Can you work these out from the model? Positions are in its coordinate system, mm. Face numbers are marked on the shaded views. Give positions to 0.01 mm unless a question says otherwise; leave off trailing zeros. Order: outer loops, then holes, each group sorted by start corner. A loop starts at its lowest first (then second) coordinate and runs counter-clockwise, first axis right, second up. Notation, with made-up numbers: (80, 61.25) - (100, 61.25) arc R27 ccw to (100, 77.25) - close; hole circle Ø7 at (3, 71.25). An arc over 180 degrees is marked (long way). Use one line per item in the form item = value. Start each with the question number.
1) Please list where these lines run through material, in increasing order: probe 1 along X at (y, z) = (51, 0); probe 2 along X at (y, z) = (15, -4.5); probe 3 along Z at (x, y) = (8, 77.5).
2) Suppose I cut it at A-A, the plane x = 0. Write out the boundary of the cut face in (y, z), and give its area (3 significant figures).
3) We'd pull the mould along Z, two halves only. Please class the marked faces 1 and 2: released by +Z, released by -Z, zero draft, split by the parting line, or undercut.
4) Suppose I cut it at B-B, the plane z = 0. Write out the boundary of the cut face in (x, y), and give its area (3 significant figures).
5) Suppose I cut it at C-C, the plane y = 51. Write out the boundary of the cut face in (x, z), and give its area (3 significant figures).
6) For pin 1 (12 mm diameter, centred on x = -18.5, y = 81, fed in from +Z); pin 2 (5 mm diameter, centred on y = 36, z = -9, fed in from -X); pin 3 (3 mm diameter, centred on x = -11, y = 34, fed in from +Z), each with a flat end and sliding along its axis, tell me the tip position at first contact or that it passes through.
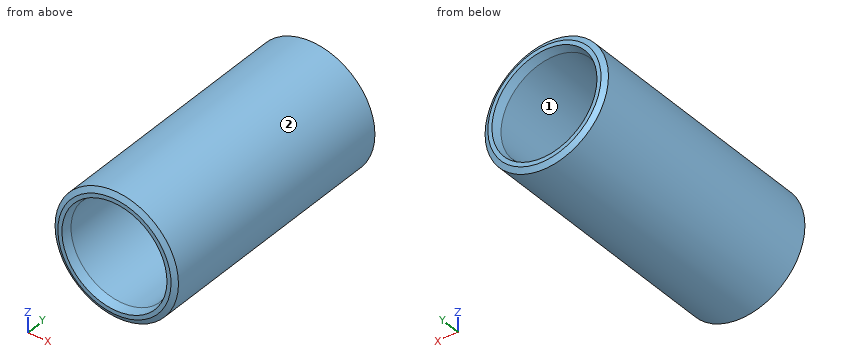
```python
from build123d import *

# Parameters (mm, degrees)
DURCHMESSER_WD_R   = 24.15
DURCHMESSER_WD_R_2 = 19.65
ROHR_DEPTH         = 100


with BuildPart() as part:
    # Durchmesser/ WD → Rohr (new body)
    with BuildSketch(Plane(origin=(0, 0, 0), x_dir=(1, 0, 0), z_dir=(0, 1, 0))):
        with Locations(Location((0, 0, 0), (0, 0, 270))):  # turned: the seam where the file's is
            Circle(DURCHMESSER_WD_R)
        with Locations(Location((0, 0, 0), (0, 0, 270))):  # turned: the seam where the file's is
            Circle(DURCHMESSER_WD_R_2, mode=Mode.SUBTRACT)
    extrude(amount=ROHR_DEPTH)

    # Fase1 → Schweißfase 1 (revolve, cut)
    with BuildSketch(Plane.XY, mode=Mode.PRIVATE) as schwei_fase_1_sk:
        Polygon((24.15, 100), (24.15, 98.845299462), (22.15, 100), align=None)
        Polygon((20.55, 100), (19.65, 100), (19.65, 96.641154273), align=None)
    revolve(schwei_fase_1_sk.sketch.rotate(Axis((0, 0, 0), (0, 1, 0)), 90), axis=Axis((0, 0, 0), (0, 1, 0)), mode=Mode.SUBTRACT)  # turned: the seam where the file's is

    # Fase2 → Schweißfase 2 (revolve, cut)
    with BuildSketch(Plane.XY, mode=Mode.PRIVATE) as schwei_fase_2_sk:
        Polygon((24.15, 0), (24.15, 1.154700538), (22.15, 0), align=None)
        Polygon((20.55, 0), (19.65, 0), (19.65, 3.358845727), align=None)
    revolve(schwei_fase_2_sk.sketch.rotate(Axis((0, 0, 0), (0, 1, 0)), 90), axis=Axis((0, 0, 0), (0, 1, 0)), mode=Mode.SUBTRACT)  # turned: the seam where the file's is


solid = part.part
```
Result sheet:
q1.probe_1 = -24.15 to -19.65, 19.65 to 24.15
q1.probe_2 = -23.73 to -19.13, 19.13 to 23.73
q1.probe_3 = -22.79 to -17.95, 17.95 to 22.79
q2.outline = (0, -22.15) - (1.15, -24.15) - (98.85, -24.15) - (100, -22.15) - (100, -20.55) - (96.64, -19.65) - (3.36, -19.65) - (0, -20.55) - close; (0, 20.55) - (3.36, 19.65) - (96.64, 19.65) - (100, 20.55) - (100, 22.15) - (98.85, 24.15) - (1.15, 24.15) - (0, 22.15) - close
q2.area = 889 mm²
q3.face_1 = undercut
q3.face_2 = split by the parting line
q4.outline = (-24.15, 1.15) - (-22.15, 0) - (-20.55, 0) - (-19.65, 3.36) - (-19.65, 96.64) - (-20.55, 100) - (-22.15, 100) - (-24.15, 98.85) - close; (19.65, 3.36) - (20.55, 0) - (22.15, 0) - (24.15, 1.15) - (24.15, 98.85) - (22.15, 100) - (20.55, 100) - (19.65, 96.64) - close
q4.area = 889 mm²
q5.outline = circle Ø48.3 at (0, 0); hole circle Ø39.3 at (0, 0)
q5.area = 619 mm²
q6.pin_1 = 20.66
q6.pin_2 = -23.26
q6.pin_3 = 22.2
